```python
from build123d import *

# Parameters (mm, degrees)
F0_W     = 63
F0_H     = 54
F0_W_2   = 59
F0_H_2   = 50
F1_DEPTH = 59
F2_DEPTH = 2
F3_W     = 1
F3_H     = 51
F4_DEPTH = 2
F5_START = 57
F5_DEPTH = 2
F6_W     = 1
F6_H     = 19
F7_DEPTH = 3


with BuildPart() as f1:
    # F0 (on Top) → F1 (new body)
    with BuildSketch(Plane.XY):
        with Locations((-808.1280109427, -717.9987351179)):
            Rectangle(F0_W, F0_H)
        with Locations((-808.1280109427, -717.9987351179)):
            Rectangle(F0_W_2, F0_H_2, mode=Mode.SUBTRACT)
    extrude(amount=F1_DEPTH)

    # F0 (on Top) → F2 (join)
    with BuildSketch(Plane.XY):
        with Locations((-808.1280109427, -717.9987351179)):
            Rectangle(F0_W_2, F0_H_2)
    extrude(amount=F2_DEPTH)

    # F3 (on face) → F4 (join)
    with BuildSketch(Plane.YZ.offset(-837.6280109427)):
        with Locations((-710.1987351179, 27.5)):
            Rectangle(F3_W, F3_H)
        with Locations((-725.8987351179, 27.5)):
            Rectangle(F3_W, F3_H)
    extrude(amount=F4_DEPTH)

    # F3 (on face) → F5 (join)
    with BuildSketch(Plane.YZ.offset(-837.6280109427).offset(F5_START)):
        with Locations((-710.1987351179, 27.5)):
            Rectangle(F3_W, F3_H)
        with Locations((-725.8987351179, 27.5)):
            Rectangle(F3_W, F3_H)
    extrude(amount=F5_DEPTH)

    # F6 (on face) → F7 (cut)
    with BuildSketch(Plane(origin=(0, -690.9987351179, 0), x_dir=(-1, 0, 0), z_dir=(0, 1, 0))):
        with Locations((823.6280109427, 29.5)):
            Rectangle(F6_W, F6_H)
        with Locations((792.6280109427, 29.5)):
            Rectangle(F6_W, F6_H)
    extrude(amount=-F7_DEPTH, mode=Mode.SUBTRACT)


solid = f1.part
```
The model under review builds one solid part; all positions refer to its coordinate system, in mm. A direction names the side the tool comes from. Give positions to 0.01 mm unless a question says otherwise; leave off trailing zeros. Write each loop counter-clockwise with the first axis right and the second up, starting at its lowest first coordinate (ties: lowest second). Pieces come first, ordered by that corner, then holes. Notation, with made-up numbers: M 50,13.5 L 106,13.5 A28 cw 106,51.5 Z; hole C 81,74.25 d3. An arc over 180 degrees is marked long. Write each question's results on one line, items separated by ' | '. Start each with the question number.
1. Mouldability with a two-part tool opening along Y and no side actions: class faces 1 (the flat face through (-809, -744.999, 29)), 2 (the flat face through (-837, -709.699, 27)), 3 (the flat face through (-776.628, -718, 29)) as released by +Y, released by -Y, zero draft, split by the parting line, or undercut.
2. For probe 1 along X at (y, z) = (-694, 30.5); probe 2 along Y at (x, z) = (-787, 6); probe 3 along X at (y, z) = (-726, 6.5), list the stretches that pass through material, from the lowest coordinate up. Write a range as [from, to].
3. Insertion check: pin 1 Ø0.8 at (x, y) = (-837, -710.5) entering from +Z; pin 2 Ø1 at (x, y) = (-823, -702) entering from +Z. Each pin has a flat end and moves straight along its axis. Give the tip position at first contact, or say it passes through.
4. We need section D-D (y = -702). Write out the cut boundary in (x, z), and give its area (3 significant figures).
5. We need section B-B (z = 45). Write out the cut boundary in (x, y), and give its area (3 significant figures).
6. We need section C-C (x = -786.5). Write out the cut boundary in (y, z), and give its area (3 significant figures).
7. For faces 4 (the flat face through (-792.128, -692, 29)), 5 (the flat face through (-837, -725.399, 27)), 6 (the flat face through (-839.628, -718, 29)), list the 3-axis set-ups (+Z, -Z, +X, -X, +Y, -Y) from which the entire face can be reached by the end or side of a thin tool; tool diameter is ignored.
Results found:
1) face 1: released by -Y | face 2: undercut | face 3: zero draft
2) probe 1: x = [-839.63, -837.63], [-778.63, -776.63] | probe 2: y = [-745, -743], [-693, -691] | probe 3: x = [-839.63, -835.63], [-780.63, -776.63]
3) pin 1: stops at z = 53 | pin 2: stops at z = 2
4) outline: M -839.63,0 L -776.63,0 L -776.63,59 L -778.63,59 L -778.63,2 L -837.63,2 L -837.63,59 L -839.63,59 Z | area: 354 mm^2
5) outline: M -839.63,-745 L -776.63,-745 L -776.63,-691 L -839.63,-691 Z; hole M -837.63,-743 L -778.63,-743 L -778.63,-726.4 L -780.63,-726.4 L -780.63,-725.4 L -778.63,-725.4 L -778.63,-710.7 L -780.63,-710.7 L -780.63,-709.7 L -778.63,-709.7 L -778.63,-693 L -837.63,-693 L -837.63,-709.7 L -835.63,-709.7 L -835.63,-710.7 L -837.63,-710.7 L -837.63,-725.4 L -835.63,-725.4 L -835.63,-726.4 L -837.63,-726.4 Z | area: 460 mm^2
6) outline: M -745,0 L -691,0 L -691,59 L -693,59 L -693,2 L -743,2 L -743,59 L -745,59 Z | area: 336 mm^2
7) face 4: +Y | face 5: +Z | face 6: +Z, -Z, -X, +Y, -Y
